```python
from build123d import *

# Parameters (mm, degrees)
F0_W     = 300
F0_H     = 110
F1_DEPTH = 30
F2_R     = 40
F3_DEPTH = 30
F4_W     = 30
F4_H     = 30
F5_DEPTH = 100
F7_DEPTH = 30
F8_SIZE  = 40


with BuildPart() as f1:
    # F0 (on Right) → F1 (new body)
    with BuildSketch(Plane.YZ):
        with Locations((150, 55)):
            Rectangle(F0_W, F0_H)
    extrude(amount=F1_DEPTH)

    # F2 (on face) → F3 (cut, through all)
    with BuildSketch(Plane.YZ.offset(30)):
        with Locations((55, 45)):
            Circle(F2_R)
        with Locations((245, 45)):
            Circle(F2_R)
    extrude(amount=-F3_DEPTH, mode=Mode.SUBTRACT)

    # F4 (on face) → F5 (join)
    with BuildSketch(Plane.YZ.offset(30)):
        with Locations((150, 95)):
            Rectangle(F4_W, F4_H)
        with Locations((150, 15)):
            Rectangle(F4_W, F4_H)
    extrude(amount=F5_DEPTH)

    # F6 (on face) → F7 (cut, through all)
    with BuildSketch(Plane(origin=(0, 165, 0), x_dir=(-1, 0, 0), z_dir=(0, 1, 0))):
        Polygon((-80, 105), (-130, 105), (-130, 80), (-30, 80), align=None)
        Polygon((-30, 30), (-130, 30), (-130, 5), (-80, 5), align=None)
    extrude(amount=-F7_DEPTH, mode=Mode.SUBTRACT)

    # F8
    f8_edges = [f1.edges().sort_by_distance(p)[0] for p in [
        (15, 0, 110),
        (15, 300, 110),
    ]]
    chamfer(f8_edges, length=F8_SIZE)


solid = f1.part
```
Verification items for the finished model (mm, model axes). A direction names the side the tool comes from. Coordinates: 2 decimals unless noted, no trailing zeros. Loops run counter-clockwise (first coordinate to the right, second up) from the corner with the lowest first, then second, coordinate; pieces in that order, holes last. Notation, with made-up numbers: (7.25, -20) - (50.25, -20) arc R21 cw to (50.25, 0) - close; hole circle Ø6 at (-22.75, 29.5). An arc over 180 degrees is marked (long way). Return JSON: item names as keys, results as strings.
1. Section check B-B, the plane y = 245. Record the boundary of the cut face in (x, z).
Established:
{"outline": "(0, 0) - (30, 0) - (30, 5) - (0, 5) - close; (0, 85) - (30, 85) - (30, 110) - (0, 110) - close"}
2. Section check C-C, the plane x = 65.5. Record the boundary of the cut face in (y, z), then the cut area to 3 significant figures.
Established:
{"outline": "(135, 0) - (165, 0) - (165, 12.25) - (135, 12.25) - close; (135, 97.75) - (165, 97.75) - (165, 110) - (135, 110) - close", "area": "735 mm2"}
3. Section check D-D, the plane y = 124. Record the boundary of the cut face in (x, z).
Established:
{"outline": "(0, 0) - (30, 0) - (30, 110) - (0, 110) - close"}
4. Mould release check, pull along Y, two halves, no side actions. Record for faces 6 (the cylindrical face through (15.21, 73.458, 9.513)), 7 (the flat face through (61, 135, 99)), 8 (the flat face through (61, 165, 99)): +Y half, -Y half, draft (parallel to the pull), parting line (faces both ways), or undercut.
Established:
{"face 6": "undercut", "face 7": "-Y half", "face 8": "+Y half"}
5. Tool access check on faces 1 (the flat face through (68, 135, 8)), 2 (the flat face through (55.4, 150.2, 17.3)), 3 (the flat face through (15, 300, 35)), 4 (the flat face through (68, 165, 8)), 5 (the flat face through (36, 149, 110)). Record the directions out of +Z, -Z, +X, -X, +Y, -Y that give a thin tool (end or side, any length) a straight path to the whole face; none if there is none.
Established:
{"face 1": "+Z, -Z, +X, -Y", "face 2": "+X, +Y, -Y", "face 3": "+Z, -Z, +X, -X, +Y", "face 4": "+Z, -Z, +X, +Y", "face 5": "+Z, +X, -X, +Y, -Y"}
6. Go/stop test with flat-tipped pins: pin 1 (3 mm diameter, centred on x = 50.5, y = 150.5, fed in from -Z); pin 2 (12 mm diameter, centred on y = 143.5, z = 37, fed in from +X); pin 3 (8 mm diameter, centred on y = 237, z = 11.5, fed in from +X). Record where each tip stops, or that it passes through.
Established:
{"pin 1": "stops at z = 0", "pin 2": "stops at x = 30", "pin 3": "passes through"}
7. Section check A-A, the plane z = 45. Record the boundary of the cut face in (x, y).
Established:
{"outline": "(0, 0) - (30, 0) - (30, 15) - (0, 15) - close; (0, 95) - (30, 95) - (30, 205) - (0, 205) - close; (0, 285) - (30, 285) - (30, 300) - (0, 300) - close"}
8. Thickness scan on L1, parallel to Z at x = 23.75, y = 245; L2, parallel to X at y = 106, z = 6; L3, parallel to Z at x = 100, y = 149.5. Record the ranges inside material, lowest first.
Established:
{"L1": "z = 0 to 5, 85 to 110", "L2": "x = 0 to 30", "L3": "z = 0 to 5, 105 to 110"}
